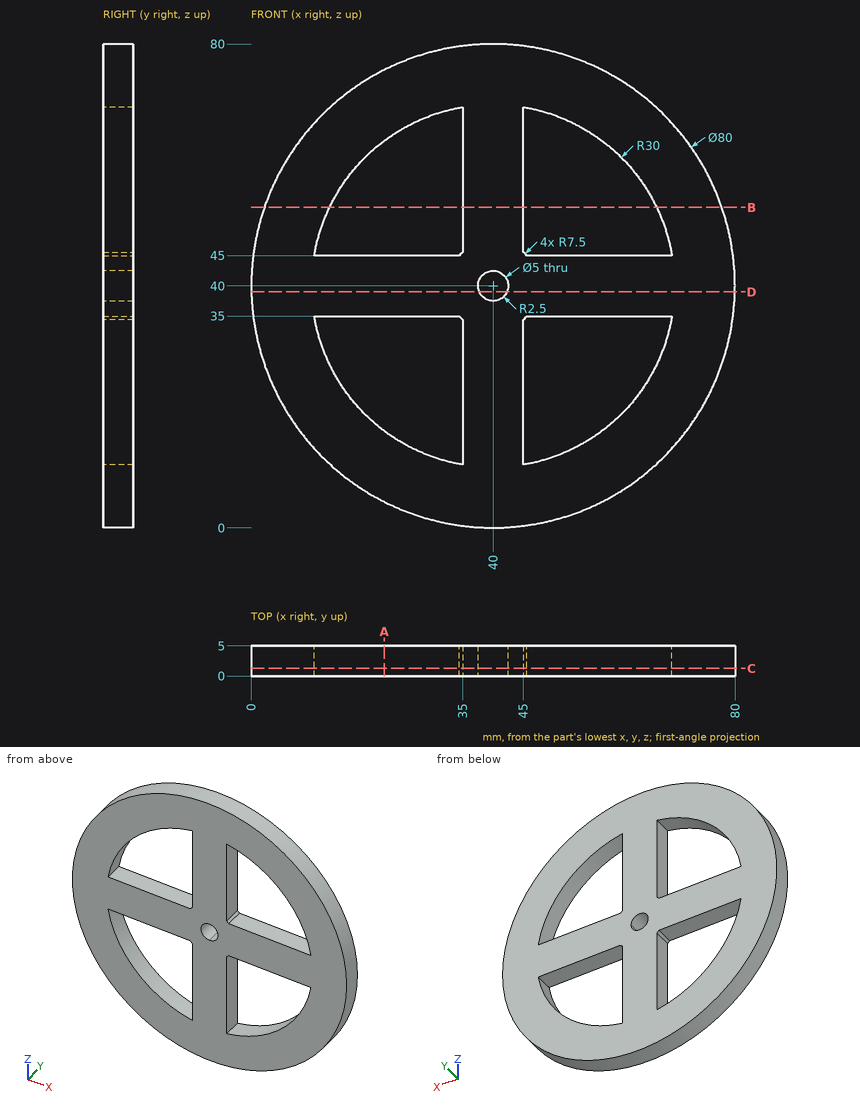
Input: dimensioned drawing with shaded views. Units: mm. Origin: part minimum x, y, z. Coordinates: 2 decimals unless noted, no trailing zeros. Loops run counter-clockwise (first coordinate to the right, second up) from the corner with the lowest first, then second, coordinate; pieces in that order, holes last. Notation, with made-up numbers: M -8,-15 L 20,-15 A25 cw 20,12 Z; hole C -25.5,5 d3. An arc over 180 degrees is marked long. One line per item, written item: value. Start each with the question number.
1) Cut plane C-C (y = 1.25). Return loops of the section in (x, z).
2) Cut plane D-D (z = 39). Return loops of the section in (x, y), then the cut area to 3 significant figures.
3) Material intervals for L1, parallel to X at y = 4.8, z = 58.5 (1 decimal); L2, parallel to Z at x = 47, y = 2.7; L3, parallel to Z at x = 30, y = 1.6, sorted ascending. Write a range as from..to.
4) Pin query (flat end, axial travel): P1, Ø6, axis at x = 45.5, z = 42.5, coming from the -Y side; P2, Ø1.5, axis at x = 25.5, y = 1.5, coming from the -Z side; P3, Ø2.5, axis at y = 1.5, z = 22, coming from the -X side; P4, Ø2.5, axis at x = 59, y = 2.5, coming from the +Z side. Return the tip coordinate at first contact, or that it passes through.
5) Cut plane B-B (z = 53). Return loops of the section in (x, y), then the cut area to 3 significant figures.
6) Cut plane A-A (x = 22). Return loops of the section in (y, z).
Evaluation:
1. outline: C 40,40 d80; hole M 10.42,35 A30 ccw 35,10.42 L 35,34.41 A7.5 cw 34.41,35 Z; hole M 10.42,45 L 34.41,45 A7.5 cw 35,45.59 L 35,69.58 A30 ccw Z; hole C 40,40 d5; hole M 45,10.42 A30 ccw 69.58,35 L 45.59,35 A7.5 cw 45,34.41 Z; hole M 45,45.59 A7.5 cw 45.59,45 L 69.58,45 A30 ccw 45,69.58 Z
2. outline: M 0.01,0 L 37.71,0 L 37.71,5 L 0.01,5 Z; M 42.29,0 L 79.99,0 L 79.99,5 L 42.29,5 Z
2. area: 377 mm^2
3. L1: 4.5..16.4, 35..45, 63.6..75.5
3. L2: 0.62..10.83, 35..45, 69.17..79.38
3. L3: 1.27..11.72, 35..45, 68.28..78.73
4. P1: y = 0
4. P2: z = 2.44
4. P3: x = 3.68
4. P4: z = 75.85
5. outline: M 2.17,0 L 12.96,0 L 12.96,5 L 2.17,5 Z; M 35,0 L 45,0 L 45,5 L 35,5 Z; M 67.04,0 L 77.83,0 L 77.83,5 L 67.04,5 Z
5. area: 158 mm^2
6. outline: M 0,4.28 L 5,4.28 L 5,16 L 0,16 Z; M 0,35 L 5,35 L 5,45 L 0,45 Z; M 0,64 L 5,64 L 5,75.72 L 0,75.72 Z
